```python
from build123d import *

# Parameters (mm, degrees)
BOSS_EXTRUDE1_DEPTH                  = 72
SKETCH2_W                            = 72
SKETCH2_H                            = 2
BOSS_EXTRUDE2_DEPTH                  = 35
BOSS_EXTRUDE2_DIRECTION_2_REACH      = 91.844
BOSS_EXTRUDE2_DIRECTION_2_END_RADIUS = 36
SKETCH3_R                            = 1.3
CUT_EXTRUDE1_DEPTH                   = 10
SKETCH4_R                            = 1.3
CUT_EXTRUDE2_DEPTH                   = 112.373246339
FILLET1_R                            = 7


with BuildPart() as part:
    # Sketch1 → Boss-Extrude1 (new body)
    with BuildSketch(Plane.XY):
        with BuildLine():
            Line((-36, 0), (-36, -35))
            Line((-36, -35), (-38, -35))
            Line((-38, -35), (-38, 0))
            ThreePointArc((-38, 0), (0, 38), (38, 0))
            Line((38, 0), (38, -35))
            Line((38, -35), (36, -35))
            Line((36, -35), (36, 0))
            ThreePointArc((36, 0), (0, 36), (-36, 0))
        make_face()
    extrude(amount=BOSS_EXTRUDE1_DEPTH)

    # Sketch2 → Boss-Extrude2 (add)
    with BuildSketch(Plane(origin=(0, 0, 0), x_dir=(1, 0, 0), z_dir=(0, 1, 0))):
        with Locations((0, -71)):
            Rectangle(SKETCH2_W, SKETCH2_H)
    extrude(amount=-BOSS_EXTRUDE2_DEPTH)

    # Boss-Extrude2 direction 2: up to this cylinder (the profile starts inside it)
    boss_extrude2_direction_2_end = Plane(origin=(0, 0, 71), z_dir=(0, 0, -1)) * Cylinder(BOSS_EXTRUDE2_DIRECTION_2_END_RADIUS, 256.688, mode=Mode.PRIVATE)
    # Sketch2 → Boss-Extrude2 direction 2 (add, up to the surface)
    with BuildSketch(Plane(origin=(0, 0, 0), x_dir=(1, 0, 0), z_dir=(0, 1, 0)), mode=Mode.PRIVATE) as boss_extrude2_direction_2_sk1:
        with Locations((0, -71)):
            Rectangle(SKETCH2_W, SKETCH2_H)
    boss_extrude2_direction_2_tool1 = extrude(boss_extrude2_direction_2_sk1.sketch, amount=BOSS_EXTRUDE2_DIRECTION_2_REACH, mode=Mode.PRIVATE) & boss_extrude2_direction_2_end
    add(boss_extrude2_direction_2_tool1.solids().sort_by_distance((0, 0, 71))[0])

    # Sketch3 → Cut-Extrude1 (cut)
    with BuildSketch(Plane.XY.offset(72)):
        with Locations((-25.9, -31)):
            Circle(SKETCH3_R)
        with Locations((25.9, -31)):
            Circle(SKETCH3_R)
    extrude(amount=-CUT_EXTRUDE1_DEPTH, mode=Mode.SUBTRACT)

    # Sketch4 → Cut-Extrude2 (cut, through all)
    with BuildSketch(Plane(origin=(38, 0, 0), x_dir=(0, 0, -1), z_dir=(1, 0, 0))):
        with Locations(Location((-11.1, -31, 0), (0, 0, 90))):
            Circle(SKETCH4_R)
    extrude(amount=-CUT_EXTRUDE2_DEPTH, mode=Mode.SUBTRACT)

    # Fillet1
    fillet1_edges = [part.edges().sort_by_distance(p)[0] for p in [
        (-37, -35, 0),
        (37, -35, 0),
    ]]
    fillet(fillet1_edges, radius=FILLET1_R)


solid = part.part
```
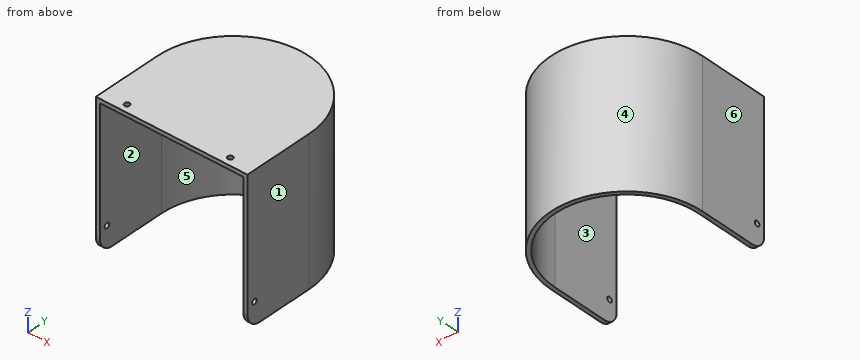
The listing builds one solid part. Answer for the finished solid, in the listing's coordinates (mm). Face numbers are marked on the shaded views. A direction names the side the tool comes from. Give positions to 0.01 mm unless a question says otherwise; leave off trailing zeros. Order: outer loops, then holes, each group sorted by start corner. A loop starts at its lowest first (then second) coordinate and runs counter-clockwise, first axis right, second up. Notation, with made-up numbers: (-10.75, 30.25) -> (-0.75, 30.25) arc R10 ccw to (-0.75, 34.25) -> close; hole circle Ø6 at (37, 42.25). An arc over 180 degrees is marked (long way). Answer as CSV lines item,"result". Start each with the question number.
Q1. Given pin 1 (3 mm diameter, centred on x = -16, z = 22, fed in from +Y); pin 2 (21.5 mm diameter, centred on x = 11.5, y = 6.5, fed in from -Z); pin 3 (2 mm diameter, centred on y = -31, z = 11.1, fed in from +X); pin 4 (1 mm diameter, centred on x = 29.5, z = 19.5, fed in from +Y), each flat-ended and moving along its own axis, determine where each tip first touches the part or whether it passes through.
Q2. Which of the six approach directions +Z, -Z, +X, -X, +Y, -Y give full straight-line access (tool end or side, diameter ignored) to the marked faces 5 and 6?
Q3. Find the intervals of material crossed by L1, parallel to X at y = -1.5, z = 68; L2, parallel to Z at x = -0.5, y = 15.5; L3, parallel to X at y = 3.5, z = 54, in increasing order.
Q4. Determine the mould class of the marked faces 1, 2, 3 and 4 for opening direction X: pulls with the +X half, pulls with the -X half, needs draft (parallel to the pull), parting line crosses it, or undercut.
Q5. A cutting plane is placed at C-C (x = -25.9). Determine the outline of the cut face in (y, z).
Q6. A cutting plane is placed at B-B (z = 11.1). Determine the outline of the cut face in (x, y), then the cut area to 3 significant figures.
Q7. A cutting plane is placed at D-D (y = -22). Determine the outline of the cut face in (x, z).
Q8. A cutting plane is placed at A-A (z = 39.5). Determine the outline of the cut face in (x, y).
Results found:
1,pin 1,"y = 35.12"
1,pin 2,"z = 70"
1,pin 3,"through"
1,pin 4,"y = 24.56"
2,face 5,"-Z, -Y"
2,face 6,"+Z, -Z, -X, +Y, -Y"
3,L1,"-38 to -36, 36 to 38"
3,L2,"70 to 72"
3,L3,"-37.84 to -35.83, 35.83 to 37.84"
4,face 1,"pulls with the +X half"
4,face 2,"undercut"
4,face 3,"undercut"
4,face 4,"parting line crosses it"
5,outline,"(-35, 70) -> (-32.3, 70) -> (-32.3, 72) -> (-35, 72) -> close; (-29.7, 70) -> (25, 70) -> (25, 0) -> (27.81, 0) -> (27.81, 72) -> (-29.7, 72) -> close"
6,outline,"(-38, -35) -> (-36, -35) -> (-36, -32.3) -> (-38, -32.3) -> close; (-38, -29.7) -> (-36, -29.7) -> (-36, 0) arc R36 cw to (36, 0) -> (36, -29.7) -> (38, -29.7) -> (38, 0) arc R38 ccw to (-38, 0) -> close; (36, -35) -> (38, -35) -> (38, -32.3) -> (36, -32.3) -> close"
6,area,"362 mm2"
7,outline,"(-38, 0) -> (-36, 0) -> (-36, 70) -> (36, 70) -> (36, 0) -> (38, 0) -> (38, 72) -> (-38, 72) -> close"
8,outline,"(-38, -35) -> (-36, -35) -> (-36, 0) arc R36 cw to (36, 0) -> (36, -35) -> (38, -35) -> (38, 0) arc R38 ccw to (-38, 0) -> close"
